Check sheet for the drawn part. Datum: minimum x, y, z corner. Units: mm. A direction names the side the tool comes from. Round coordinates to 2 decimals unless told otherwise and drop trailing zeros. Write each loop counter-clockwise with the first axis right and the second up, starting at its lowest first coordinate (ties: lowest second). Pieces come first, ordered by that corner, then holes. Notation, with made-up numbers: M 53.25,-8 L 88.25,-8 A20 ccw 88.25,22 Z; hole C 14.25,43 d11. An arc over 180 degrees is marked long. Put each result on its own line as item: value.
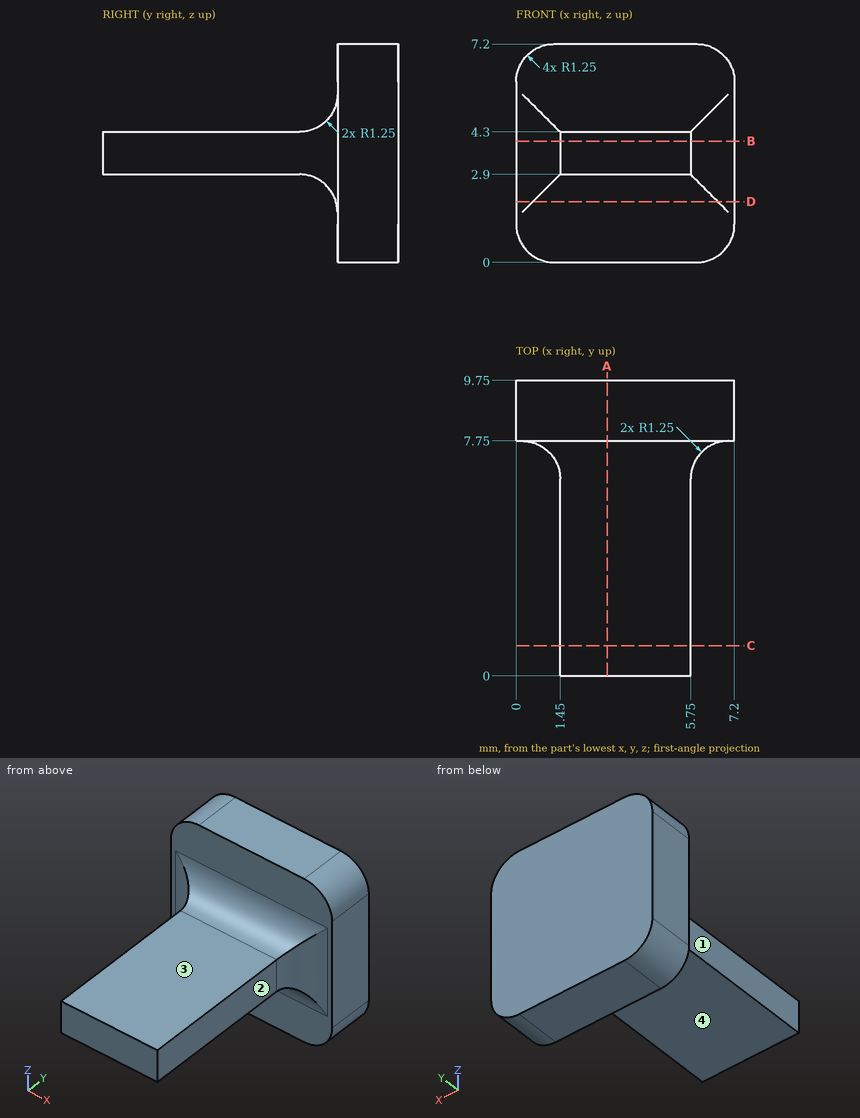
1. Cross-section at A-A (x = 3). Enter the section's corners in (y, z).
Computed values:
outline: M 0,2.9 L 6.5,2.9 A1.25 cw 7.75,1.65 L 7.75,0 L 9.75,0 L 9.75,7.2 L 7.75,7.2 L 7.75,5.55 A1.25 cw 6.5,4.3 L 0,4.3 Z
2. Cross-section at D-D (z = 2). Enter the section's corners in (x, y).
Computed values:
outline: M 0,7.75 L 0.2,7.75 A1.25 cw 0.55,7.7 L 6.65,7.7 A1.25 cw 7,7.75 L 7.2,7.75 L 7.2,9.75 L 0,9.75 Z
3. Cross-section at B-B (z = 4). Enter the section's corners in (x, y).
Computed values:
outline: M 0,7.75 L 0.2,7.75 A1.25 cw 1.45,6.5 L 1.45,0 L 5.75,0 L 5.75,6.5 A1.25 cw 7,7.75 L 7.2,7.75 L 7.2,9.75 L 0,9.75 Z
4. Scan lines: probe 1 along Y at (x, z) = (3.5, 1); probe 2 along Z at (x, y) = (5.5, 4.75); probe 3 along Y at (x, z) = (6.25, 2). Record each from-to range of solid material in increasing order.
Computed values:
probe 1: y = 7.75 to 9.75
probe 2: z = 2.9 to 4.3
probe 3: y = 7.7 to 9.75
5. Depth check by flat-ended pin: pin 1 Ø3 at (x, y) = (3.5, 1) entering from +Z; pin 2 Ø1.5 at (y, z) = (1, 5) entering from -X; pin 3 Ø4 at (x, y) = (5, 6.5) entering from -Z; pin 4 Ø2 at (x, y) = (5, 6.5) entering from -Z. Enter the tip coordinate at first touch or a pass-through.
Computed values:
pin 1: stops at z = 4.3
pin 2: stops at x = 1.45
pin 3: stops at z = 0
pin 4: stops at z = 2.4
6. Access from +Z, -Z, +X, -X, +Y, -Y to the whole of each face (thin tool, end or side, straight path). Record for the marked faces 1, 2, 3 and 4.
Computed values:
face 1: +Z, -Z, -X, -Y
face 2: +Z, -Z, +X, -Y
face 3: +Z, +X, -X, -Y
face 4: -Z, +X, -X, -Y
7. Cross-section at C-C (y = 1). Enter the section's corners in (x, z), then the cut area to 3 significant figures.
Computed values:
outline: M 1.45,2.9 L 5.75,2.9 L 5.75,4.3 L 1.45,4.3 Z
area: 6.02 mm2
